Read the model definition and answer for the solid it produces. Units are mm, in the model's axes. A direction names the side the tool comes from. Round coordinates to 2 decimals unless told otherwise and drop trailing zeros. Loops run counter-clockwise (first coordinate to the right, second up) from the corner with the lowest first, then second, coordinate; pieces in that order, holes last. Notation, with made-up numbers: M 84.5,-32 L 119.5,-32 A14 ccw 119.5,-20 Z; hole C 63.25,9 d5. An arc over 180 degrees is marked long. Answer as CSV lines item,"result".
```python
from build123d import *

# Parameters (mm, degrees)
F0_R     = 15.875
F0_R_2   = 10.16
F1_DEPTH = 9.525
F2_DEPTH = 15.875
F3_SIZE2 = 1.5748
F3_SIZE  = 6.35
F4_SIZE  = 5.08
F5_R     = 0.508


with BuildPart() as f1:
    # F0 (on Top) → F1 (new body)
    with BuildSketch(Plane.XY):
        Circle(F0_R)
        Circle(F0_R_2, mode=Mode.SUBTRACT)
        Circle(F0_R_2)
    extrude(amount=-F1_DEPTH)

    # F0 (on Top) → F2 (join)
    with BuildSketch(Plane.XY):
        Circle(F0_R_2)
    extrude(amount=F2_DEPTH)

    # F3
    f3_edges = [f1.edges().sort_by_distance(p)[0] for p in [
        (-10.16, 0, 15.875),
    ]]
    f3_side = f1.faces().sort_by_distance((-10.16, 0, 7.9375))[0]
    chamfer(f3_edges, length=F3_SIZE, length2=F3_SIZE2, reference=f3_side)

    # F4
    f4_edges = [f1.edges().sort_by_distance(p)[0] for p in [
        (-15.875, 0, -9.525),
    ]]
    chamfer(f4_edges, length=F4_SIZE)

    # F5
    f5_edges = [f1.edges().sort_by_distance(p)[0] for p in [
        (-15.875, 0, 0),
        (-15.875, 0, -4.445),
        (-10.795, 0, -9.525),
    ]]
    fillet(f5_edges, radius=F5_R)


solid = f1.part
```
1) Determine the mould class of faces 1 (the cylindrical face through (15.14, 4.77, -2.35)), 2 (the flat face through (0, 0, -9.525)) for opening direction X: released by +X, released by -X, zero draft, split by the parting line, or undercut.
Evaluation:
face 1,"split by the parting line"
face 2,"zero draft"
2) A tool of negligible diameter and unlimited length cuts with its end or side. For faces 3 (the cylindrical face through (-1.323, 10.074, 4.696)), 4 (the flat face through (0, 0, 15.875)), from which of +Z, -Z, +X, -X, +Y, -Y can it reach the whole face along a straight path? Write none if from no direction.
Evaluation:
face 3,"+Z"
face 4,"+Z, +X, -X, +Y, -Y"
3) Find section A-A, the plane z = 2. Give the vertices of the cut face in (x, y).
Evaluation:
outline,"C 0,0 d20.32"
4) Each of these flat-tipped pins is pushed along its axis until it touches: P1, Ø8, axis at y = 11, z = 1.5, coming from the +X side; P2, Ø10, axis at y = 12, z = -5.5, coming from the +X side; P3, Ø5, axis at y = 6.5, z = 7.5, coming from the +X side. Where does it stop, or does it pass through?
Evaluation:
P1,"stops at x = 13.99"
P2,"stops at x = 14.17"
P3,"stops at x = 9.34"
5) Find section B-B, the plane z = -7.5. Give the vertices of the cut face in (x, y).
Evaluation:
outline,"C 0,0 d25.64"
6) Straight lines are drawn through the part: line 1 (Z direction, x = -10, y = 2.5) (3 decimals); line 2 (Y direction, x = 3, z = 8.75); line 3 (X direction, y = -8, z = 12.5). For each, find the intervals that lie inside material, in ascending order.
Evaluation:
line 1,"z = -9.525 to 0"
line 2,"y = -9.71 to 9.71"
line 3,"x = -4.98 to 4.98"
